Check sheet for the modelled part. Datum: model origin and axes. Units: mm. A direction names the side the tool comes from. Round coordinates to 2 decimals unless told otherwise and drop trailing zeros. Order: outer loops, then holes, each group sorted by start corner. A loop starts at its lowest first (then second) coordinate and runs counter-clockwise, first axis right, second up. Notation, with made-up numbers: (-10.75, 66) -> (39.25, 66) arc R13 ccw to (39.25, 90) -> close; hole circle Ø2 at (0, 65). An arc over 180 degrees is marked (long way). Answer in a Markdown table with one row per item.
from build123d import *

# Parameters (mm, degrees)
F0_W     = 50.8
F0_H     = 50.8
F1_DEPTH = 25.4
F2_R     = 19.05
F3_DEPTH = 25.4
F5_DEPTH = 25.4


with BuildPart() as f1:
    # F0 (on Front) → F1 (new body)
    with BuildSketch(Plane.XZ):
        Rectangle(F0_W, F0_H)
    extrude(amount=F1_DEPTH)

    # F2 (on face) → F3 (join)
    with BuildSketch(Plane.XZ.offset(25.4)):
        Circle(F2_R)
    extrude(amount=F3_DEPTH)

    # F4 (on face) → F5 (join)
    with BuildSketch(Plane.XZ.offset(50.8)):
        Polygon((11.341736, -11.43), (0, 11.43), (-11.341736, -11.43), align=None)
    extrude(amount=F5_DEPTH)


solid = f1.part
Item 1: Depth check by flat-ended pin: P1, Ø25, axis at x = -0.5, y = -69.5, coming from the -Z side; P2, Ø6, axis at y = -40, z = -20, coming from the +X side; P3, Ø4, axis at x = -12, z = 10.5, coming from the -Y side. Enter the tip coordinate at first touch or a pass-through.
Result sheet:
| item | result |
|---|---|
| P1 | stops at z = -11.43 |
| P2 | stops at x = 8.6 |
| P3 | stops at y = -50.8 |
Item 2: Cross-section at B-B (z = -4). Record the boundary of the cut face in (x, y).
Result sheet:
| item | result |
|---|---|
| outline | (-25.4, -25.4) -> (-18.63, -25.4) -> (-18.63, -50.8) -> (-7.66, -50.8) -> (-7.66, -76.2) -> (7.66, -76.2) -> (7.66, -50.8) -> (18.63, -50.8) -> (18.63, -25.4) -> (25.4, -25.4) -> (25.4, 0) -> (-25.4, 0) -> close |
Item 3: Scan lines: line 1 (Y direction, x = -0.5, z = -18); line 2 (Y direction, x = -15, z = 18); line 3 (Z direction, x = 0.5, y = -33.5). Record each from-to range of solid material in increasing order. Write a range as [from, to].
Result sheet:
| item | result |
|---|---|
| line 1 | y = [-50.8, 0] |
| line 2 | y = [-25.4, 0] |
| line 3 | z = [-19.04, 19.04] |
Item 4: Cross-section at D-D (z = -20). Record the boundary of the cut face in (x, y), and give its area (3 significant figures).
Result sheet:
| item | result |
|---|---|
| outline | (-25.4, -25.4) -> (25.4, -25.4) -> (25.4, 0) -> (-25.4, 0) -> close |
| area | 1,290 mm^2 |
Item 5: Cross-section at C-C (y = -48). Record the boundary of the cut face in (x, z), and give its area (3 significant figures).
Result sheet:
| item | result |
|---|---|
| outline | circle Ø38.1 at (0, 0) |
| area | 1,140 mm^2 |
Item 6: Cross-section at A-A (y = -63). Record the boundary of the cut face in (x, z).
Result sheet:
| item | result |
|---|---|
| outline | (-11.34, -11.43) -> (11.34, -11.43) -> (0, 11.43) -> close |
Item 7: Set-up check for faces 1 (the flat face through (-5.59, -63.32, 0.16)), 2 (the flat face through (11, -25.4, 17)), 3 (the flat face through (-25.4, -13, 0)), 4 (the flat face through (0, -63, -11.43)), 5 (the flat face through (5.75, -63.32, -0.16)): record each of +Z, -Z, +X, -X, +Y, -Y from which the full face is reachable in a straight line by a thin tool's end or side.
Result sheet:
| item | result |
|---|---|
| face 1 | +Z, -X, -Y |
| face 2 | -Y |
| face 3 | +Z, -Z, -X, +Y, -Y |
| face 4 | -Z, +X, -X, -Y |
| face 5 | +Z, +X, -Y |
